```python
from build123d import *

# Parameters (mm, degrees)
BASENUTSKE_R       = 5.25
BASENUT_DEPTH      = 4
SKETCH4_W          = 0.4064
SKETCH4_H          = 11.392304845
SKETCH6_R          = 6
CUT_EXTRUDE1_DEPTH = 10


with BuildPart() as part:
    # BaseNutSke → BaseNut (new body)
    with BuildSketch(Plane.XY):
        Polygon((9, 5.196152423), (9, -5.196152423), (0, -10.392304845), (-9, -5.196152423), (-9, 5.196152423), (0, 10.392304845), align=None)
        Circle(BASENUTSKE_R, mode=Mode.SUBTRACT)
    extrude(amount=-BASENUT_DEPTH)

    # Sketch4 → Bearing-Face (revolve, cut)
    with BuildSketch(Plane(origin=(0, 0, 0), x_dir=(0, 0, -1), z_dir=(1, 0, 0))):
        with Locations((3.7968, 14.696152423)):
            Rectangle(SKETCH4_W, SKETCH4_H)
        Polygon((0, 9), (-10, 9), (-10, 20.392304845), (0.803847577, 20.392304845), (0.803847577, 10.392304845), align=None)
    revolve(axis=Axis((0, 0, 0), (0, 0, -1)), mode=Mode.SUBTRACT)

    # Sketch3 → Double-Chamfer (revolve, cut)
    with BuildSketch(Plane(origin=(0, 0, 0), x_dir=(0, 0, -1), z_dir=(1, 0, 0))):
        Polygon((4, 9), (3.196152423, 10.392304845), (3.196152423, 20.392304845), (14, 20.392304845), (14, 9), align=None)
        Polygon((1.201295155, 20.392304845), (-9.602552423, 20.392304845), (-9.602552423, 9), (0.397447577, 9), (1.201295155, 10.392304845), align=None)
    revolve(axis=Axis((0, 0, 0), (0, 0, -1)), mode=Mode.SUBTRACT)

    # Sketch5 → EndChamfer (revolve, cut)
    with BuildSketch(Plane(origin=(0, 0, 0), x_dir=(0, 0, -1), z_dir=(1, 0, 0))):
        Polygon((3.9746, 6.8375), (2.751862586, 5.09125), (4.0254, 5.09125), (4.0254, 6.8375), align=None)
        Polygon((-0.0508, 6.8375), (0, 6.8375), (1.222737414, 5.09125), (-0.0508, 5.09125), align=None)
    revolve(axis=Axis((0, 0, -25.037505729), (0, 0, -1)), mode=Mode.SUBTRACT)

    # ThdSchSke → ThreadSchematic (revolve, cut)
    with BuildSketch(Plane(origin=(0, 0, 0), x_dir=(1, 0, 0), z_dir=(0, 1, 0))):
        Polygon((-6.8375, 0.0254), (-5.25, 1.136979467), (-2.625, 1.136979467), (-2.625, -1.086179467), (-5.25, -1.086179467), align=None)
    revolve(axis=Axis((0, 0, -3.175), (0, 0, 1)), mode=Mode.SUBTRACT)

    # Sketch6 → Cut-Extrude1 (cut)
    with BuildSketch(Plane.XY):
        Circle(SKETCH6_R)
    extrude(amount=-CUT_EXTRUDE1_DEPTH, mode=Mode.SUBTRACT)


solid = part.part
```
Verification items for the finished model (mm, model axes). A direction names the side the tool comes from. Coordinates: 2 decimals unless noted, no trailing zeros. Write each loop counter-clockwise with the first axis right and the second up, starting at its lowest first coordinate (ties: lowest second). Pieces come first, ordered by that corner, then holes. Notation, with made-up numbers: (33, 81.5) - (75, 81.5) arc R21 ccw to (75, 100.5) - close; hole circle Ø2 at (-25.5, -3). An arc over 180 degrees is marked (long way). One line per question, with ' | ' between items. Start each with the question number.
1. Material ranges on line 1 along X through (y, z) = (0, -2.4); line 2 along Y through (x, z) = (2.5, -3.5); line 3 along Y through (x, z) = (4.5, -0.3), recorded low to high.
2. Section check A-A (z = -1.7). Enter the section's corners in (x, y), plus the area to 3 significant figures.
3. Draft check along Y on faces 1 (the flat face through (0, -9.2, -3.594)), 2 (the cylindrical face through (-1.301, -5.857, -1.981)), 3 (the conical face through (8.076, 4.689, -0.593)). Enter one of: released by +Y, released by -Y, zero draft, split by the parting line, or undercut.
4. Access from +Z, -Z, +X, -X, +Y, -Y to the whole of each face (thin tool, end or side, straight path). Record for faces 4 (the flat face through (-8.1, 4.5, -3.594)), 5 (the flat face through (8.1, 4.5, -3.594)), 6 (the conical face through (-8.099, 4.649, -0.593)), 7 (the flat face through (-4.56, 7.76, -1.97)), 8 (the cylindrical face through (2.703, 8.584, -0.202)).
5. Gauge pin test, flat ends, axial feed: P1, Ø1, axis at y = 6.5, z = -1.5, coming from the +X side; P2, Ø3, axis at x = 4.5, y = 1.5, coming from the +Z side. Record the tip position at first contact, or that the pin passes through.
Computed values:
1) line 1: -9 to -6, 6 to 9 | line 2: -8.95 to -5.63, 5.63 to 8.95 | line 3: -7.79 to -4.61, 4.61 to 7.79
2) outline: (-9, -5.2) - (0, -10.39) - (9, -5.2) - (9, 5.2) - (0, 10.39) - (-9, 5.2) - close; hole circle Ø12 at (0, 0) | area: 167 mm²
3) face 1: zero draft | face 2: undercut | face 3: released by +Y
4) face 4: -Z, -X, +Y | face 5: -Z, +X, +Y | face 6: +Z, -X, +Y | face 7: +Z, -Z, -X, +Y | face 8: +Z
5) P1: x = 7.61 | P2: z = -0.44
